The model under review builds one solid part; all positions refer to its coordinate system, in mm. A direction names the side the tool comes from. Coordinates: 2 decimals unless noted, no trailing zeros. Loops run counter-clockwise (first coordinate to the right, second up) from the corner with the lowest first, then second, coordinate; pieces in that order, holes last. Notation, with made-up numbers: M -23,71 L 10,71 A30 cw 10,97 Z; hole C 75.5,20.25 d9. An arc over 180 degrees is marked long. Use CSV: the item, a comma, the result in double quotes. Start each with the question number.
1. For L1, parallel to Y at x = -2.5, z = -3.75; L2, parallel to Y at x = 3.5, z = 2; L3, parallel to X at y = 9, z = 3, list the stretches that pass through material, from the lowest coordinate up.
2. Draft analysis for pull direction Y (two halves, no side actions). For faces 1 (the flat face through (0, 0, 0)), 2 (the flat face through (0, 60, 0)), 3 (the cylindrical face through (3.905, 56.993, 0.867)), 4 (the cylindrical face through (-4.88, 29.63, -1.08)), state which applies: +Y half, -Y half, draft (parallel to the pull), parting line (faces both ways), or undercut.
3. Tool access review of faces 5 (the cylindrical face through (-3.905, 2.993, 0.867)), 6 (the cylindrical face through (-4.88, 58.24, -1.08)): name each direction out of +Z, -Z, +X, -X, +Y, -Y from which nothing blocks a thin tool from reaching the whole face with its end or side.
4. Add section A-A, the plane y = 4. Write out the cut boundary in (x, z).
5. Clearance check with flat-ended pins moving along their axes: P1, Ø1.5, axis at x = 2.5, z = -2, coming from the -Y side; P2, Ø1.5, axis at y = 26.5, z = 1.5, coming from the +X side. State where each tip first meets the part, or that it passes through.
from build123d import *

# Parameters (mm, degrees)
SKETCH1_R           = 5
BOSS_EXTRUDE1_DEPTH = 60
CHAMFER1_SIZE       = 1
CUT_EXTRUDE1_START  = -2.5
SKETCH2_R           = 7.5
SKETCH2_R_2         = 4
CUT_EXTRUDE1_DEPTH  = 1
CUT_EXTRUDE2_START  = -3.5
SKETCH3_R           = 7.5
SKETCH3_R_2         = 4
CUT_EXTRUDE2_DEPTH  = 1


with BuildPart() as part:
    # Sketch1 → Boss-Extrude1 (new body)
    with BuildSketch(Plane(origin=(0, 0, 0), x_dir=(1, 0, 0), z_dir=(0, 1, 0))):
        with Locations(Location((0, 0, 0), (0, 0, 270))):
            Circle(SKETCH1_R)
    extrude(amount=BOSS_EXTRUDE1_DEPTH)

    # Chamfer1
    chamfer1_edges = [part.edges().sort_by_distance(p)[0] for p in [
        (0, 0, -5),
        (0, 60, -5),
    ]]
    chamfer(chamfer1_edges, length=CHAMFER1_SIZE)

    # Sketch2 → Cut-Extrude1 (cut)
    with BuildSketch(Plane.XZ.offset(CUT_EXTRUDE1_START)):
        Circle(SKETCH2_R)
        with Locations(Location((0, 0, 0), (0, 0, 270))):
            Circle(SKETCH2_R_2, mode=Mode.SUBTRACT)
    extrude(amount=-CUT_EXTRUDE1_DEPTH, mode=Mode.SUBTRACT)

    # Sketch3 → Cut-Extrude2 (cut)
    with BuildSketch(Plane(origin=(0, 60, 0), x_dir=(1, 0, 0), z_dir=(0, 1, 0)).offset(CUT_EXTRUDE2_START)):
        Circle(SKETCH3_R)
        with Locations(Location((0, 0, 0), (0, 0, 90))):
            Circle(SKETCH3_R_2, mode=Mode.SUBTRACT)
    extrude(amount=CUT_EXTRUDE2_DEPTH, mode=Mode.SUBTRACT)


solid = part.part
Computed:
1,L1,"y = 0.51 to 2.5, 3.5 to 56.5, 57.5 to 59.49"
1,L2,"y = 0.03 to 2.5, 3.5 to 56.5, 57.5 to 59.97"
1,L3,"x = -4 to 4"
2,face 1,"-Y half"
2,face 2,"+Y half"
2,face 3,"undercut"
2,face 4,"draft"
3,face 5,"none"
3,face 6,"+Y, -Y"
4,outline,"C 0,0 d10"
5,P1,"stops at y = 0"
5,P2,"stops at x = 4.94"
